from build123d import *

# Parameters (mm, degrees)
SKETCH1_R           = 4.7625
BOSS_EXTRUDE1_DEPTH = 20.32
SKETCH2_W           = 3.175
SKETCH2_H           = 12.7
BOSS_EXTRUDE2_DEPTH = 19.05
CUT_EXTRUDE1_DEPTH  = 37.015654929
SKETCH4_R           = 3.175
CUT_EXTRUDE2_DEPTH  = 37.015654929
FILLET1_R           = 2.54


with BuildPart() as part:
    # Sketch1 → Boss-Extrude1 (new body)
    with BuildSketch(Plane.XY):
        with Locations((-80.781588965, -8.89)):
            Circle(SKETCH1_R)
    extrude(amount=BOSS_EXTRUDE1_DEPTH)

    # Sketch2 → Boss-Extrude2 (add)
    with BuildSketch(Plane(origin=(0, -10, 0), x_dir=(1, 0, 0), z_dir=(0, 1, 0))):
        with Locations((-80.781588965, -10.16)):
            Rectangle(SKETCH2_W, SKETCH2_H)
    extrude(amount=-BOSS_EXTRUDE2_DEPTH)

    # Sketch3 → Cut-Extrude1 (cut, through all)
    with BuildSketch(Plane.ZY.offset(82.369088965)):
        with BuildLine():
            ThreePointArc((16.51, -22.7), (14.650128061, -27.190128061), (10.16, -29.05))
            Line((10.16, -29.05), (16.51, -29.05))
            Line((16.51, -29.05), (16.51, -22.7))
        make_face()
        with BuildLine():
            ThreePointArc((10.16, -29.05), (5.669871939, -27.190128061), (3.81, -22.7))
            Line((3.81, -22.7), (3.81, -29.05))
            Line((3.81, -29.05), (10.16, -29.05))
        make_face()
    extrude(amount=-CUT_EXTRUDE1_DEPTH, mode=Mode.SUBTRACT)

    # Sketch4 → Cut-Extrude2 (cut, through all)
    with BuildSketch(Plane.ZY.offset(82.369088965)):
        with Locations((10.16, -22.7)):
            Circle(SKETCH4_R)
    extrude(amount=-CUT_EXTRUDE2_DEPTH, mode=Mode.SUBTRACT)

    # Fillet1
    fillet1_edges = [part.edges().sort_by_distance(p)[0] for p in [
        (-82.369088965, -13.380128061, 10.16),
        (-79.194088965, -13.380128061, 10.16),
    ]]
    fillet(fillet1_edges, radius=FILLET1_R)


solid = part.part
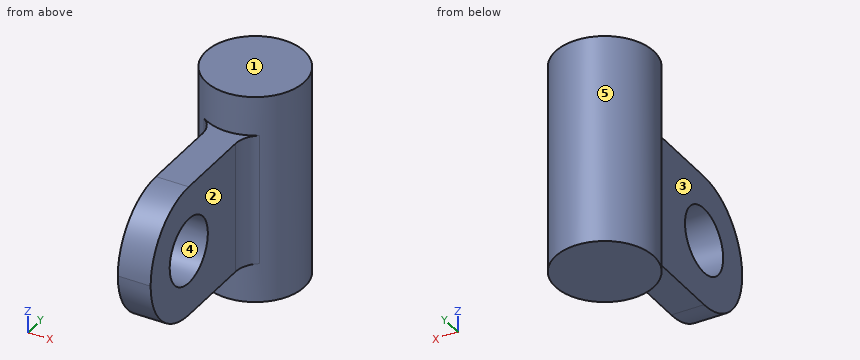
Input: part model. Units: mm. Frame: model coordinates. Face numbers are marked on the shaded views. A direction names the side the tool comes from. Coordinates: 2 decimals unless noted, no trailing zeros. Loops run counter-clockwise (first coordinate to the right, second up) from the corner with the lowest first, then second, coordinate; pieces in that order, holes last. Notation, with made-up numbers: (4.5, -10) -> (13.5, -10) arc R24 ccw to (13.5, 2) -> close; hole circle Ø1 at (7, 28). An arc over 180 degrees is marked (long way). One line per item, written item: value.
(1) Cut plane B-B (y = -18.75). Output: boundary loops of the cut face in (x, z).
Answer below:
outline: (-82.37, 3.81) -> (-79.19, 3.81) -> (-79.19, 16.51) -> (-82.37, 16.51) -> close
(2) Cut plane C-C (x = -78.75). Output: boundary loops of the cut face in (y, z), then the cut area to 3 significant figures.
Answer below:
outline: (-13.48, 3.81) -> (-13.2, 3.81) -> (-13.2, 0) -> (-4.58, 0) -> (-4.58, 20.32) -> (-13.2, 20.32) -> (-13.2, 16.51) -> (-13.48, 16.51) -> close
area: 179 mm2
(3) Pin query (flat end, axial travel): pin 1 Ø1.6 at (x, y) = (-80, -19) entering from +Z; pin 2 Ø4 at (y, z) = (-13.5, 6.5) entering from +X; pin 3 Ø4 at (y, z) = (-22.7, 10.16) entering from -X; pin 4 Ø2 at (x, z) = (-77.5, 17) entering from -Y. Return the tip coordinate at first contact, or that it passes through.
Answer below:
pin 1: stops at z = 16.51
pin 2: stops at x = -76.8
pin 3: passes through
pin 4: stops at y = -13.07
(4) Draft query along Y for the marked faces 3, 4 and 5. Return one class per face: pulls with the +Y half, pulls with the -Y half, needs draft (parallel to the pull), parting line crosses it, or undercut.
Answer below:
face 3: needs draft
face 4: undercut
face 5: parting line crosses it
(5) Cut plane D-D (z = 12.5). Output: boundary loops of the cut face in (x, y) (1 decimal).
Answer below:
outline: (-83.5, -12.8) arc R2.5 cw to (-82.4, -14.9) -> (-82.4, -20.6) -> (-79.2, -20.6) -> (-79.2, -14.9) arc R2.5 cw to (-78.1, -12.8) arc R4.8 ccw (long way) to start; (-82.4, -28.6) -> (-79.2, -28.6) -> (-79.2, -24.8) -> (-82.4, -24.8) -> close
(6) Set-up query: the marked faces 1 and 2. Return all of +Z, -Z, +X, -X, +Y, -Y with unobstructed straight access to the full face (end or side cutting, diameter ignored); none if empty.
Answer below:
face 1: +Z, +X, -X, +Y, -Y
face 2: +Z, -Z, +X, -Y
(7) Cut plane A-A (z = 9.5). Output: boundary loops of the cut face in (x, y) (1 decimal).
Answer below:
outline: (-83.5, -12.8) arc R2.5 cw to (-82.4, -14.9) -> (-82.4, -19.6) -> (-79.2, -19.6) -> (-79.2, -14.9) arc R2.5 cw to (-78.1, -12.8) arc R4.8 ccw (long way) to start; (-82.4, -29) -> (-79.2, -29) -> (-79.2, -25.8) -> (-82.4, -25.8) -> close
(8) Ray query, line 1 along Y through (x, z) = (-80.95, 10.16) (3 decimals); line 2 along X through (y, z) = (-24, 13.25); line 3 along Z through (x, y) = (-79.25, -19.25). Return the intervals inside material, ascending.
Answer below:
line 1: y = -29.05 to -25.875, -19.525 to -4.13
line 2: x = -82.37 to -79.19
line 3: z = 3.81 to 16.51
